Read the model definition and answer for the solid it produces. Units are mm, in the model's axes. Coordinates: 2 decimals unless noted, no trailing zeros. Order: outer loops, then holes, each group sorted by start corner. A loop starts at its lowest first (then second) coordinate and runs counter-clockwise, first axis right, second up. Notation, with made-up numbers: M -5.5,85 L 26.5,85 A31 cw 26.5,118 Z; hole C 2,85.5 d4. An arc over 180 degrees is marked long. Use a Markdown table: item, result. Add a question column.
1) Find the intervals of material crossed by probe 1 along Y at (x, z) = (72, 0.25); probe 2 along X at (y, z) = (11, 0.8); probe 3 along X at (y, z) = (42.5, 0.75), in increasing order. Write a range as [from, to].
2) This flat-tipped pin is pushed along its axis until it touches: pin 1 Ø0.5 at (y, z) = (6.5, 0.5) entering from -X. Where does it stop, or does it pass through?
3) Find section B-B on y = 12.5. Write down the section's boundary in (x, z), plus the area to 3 significant figures.
4) Find section A-A on z = 0.7. Write down the section's boundary in (x, y), plus the area to 3 significant figures.
5) Find section C-C on y = 35. Write down the section's boundary in (x, z), plus the area to 3 significant figures.
Autodesk Fusion 360 part; units mm, degrees
sketch "Sketch1" plane through (0, 0, 0) normal (0, 0, 1) x (1, 0, 0)
  line L0 (3.6667, 44.4476) -> (76.5667, 44.4476)
  line L1 (76.5667, 44.4476) -> (76.5667, 2.6476)
  line L2 (76.5667, 2.6476) -> (3.6667, 2.6476)
  line L3 (3.6667, 2.6476) -> (3.6667, 44.4476)
  line L4 (3.6667, 23.5476) -> (76.5667, 23.5476) construction
  line L5 (3.6667, 28.5476) -> (-0.0333, 28.5476)
  line L6 (-1.3333, 27.2476) -> (-1.3333, 19.8476)
  line L7 (-0.0333, 18.5476) -> (3.6667, 18.5476)
  line L8 (3.6667, 18.5476) -> (3.6667, 28.5476)
  arc A0 (-0.0333, 28.5476) -> (-1.3333, 27.2476) centre (-0.0333, 27.2476) ccw
  arc A1 (-1.3333, 19.8476) -> (-0.0333, 18.5476) centre (-0.0333, 19.8476) ccw
  line L9 (76.5667, 2.6476) -> (67.5667, 2.6476)
  line L10 (67.5667, 2.6476) -> (67.5667, 18.6476)
  line L11 (67.5667, 18.6476) -> (76.5667, 18.6476)
  line L12 (76.5667, 18.6476) -> (76.5667, 2.6476)
  point P0 (-1.3333, 28.5476)
  point P1 (-1.3333, 18.5476)
  dimension "d1" = 72.9
  dimension "d2" = 41.8
  dimension "d7" = 10
  dimension "d8" = 5
  dimension "d9" = 1.3
  dimension "d10" = 16
  dimension "d11" = 9
extrude "Extrude1" add sketch "Sketch1" along normal blind 1 contours L0 L1 L2 L3 L8 L10 L11 | L3 L5 L6 L7 L8 A0 A1
Check result:
| question | item | result |
|---|---|---|
| 1 | probe 1 | y = [18.65, 44.45] |
| 1 | probe 2 | x = [3.67, 67.57] |
| 1 | probe 3 | x = [3.67, 76.57] |
| 2 | pin 1 | stops at x = 3.67 |
| 3 | outline | M 3.67,0 L 67.57,0 L 67.57,1 L 3.67,1 Z |
| 3 | area | 63.9 mm2 |
| 4 | outline | M -1.33,19.85 A1.3 ccw -0.03,18.55 L 3.67,18.55 L 3.67,2.65 L 67.57,2.65 L 67.57,18.65 L 76.57,18.65 L 76.57,44.45 L 3.67,44.45 L 3.67,28.55 L -0.03,28.55 A1.3 ccw -1.33,27.25 Z |
| 4 | area | 2,950 mm2 |
| 5 | outline | M 3.67,0 L 76.57,0 L 76.57,1 L 3.67,1 Z |
| 5 | area | 72.9 mm2 |
